```python
from build123d import *

# Parameters (mm, degrees)
F0_R     = 133.35
F1_DEPTH = 355.6
F2_W     = 101.6
F2_H     = 203.2
F3_DEPTH = 304.8
F4_R     = 127
F5_DEPTH = 355.601


with BuildPart() as f1:
    # F0 (on Front) → F1 (new body)
    with BuildSketch(Plane.XZ):
        Circle(F0_R)
    extrude(amount=F1_DEPTH)

    # F2 (on Top) → F3 (join)
    with BuildSketch(Plane.XY):
        with Locations((0, -203.2)):
            Rectangle(F2_W, F2_H)
    extrude(amount=F3_DEPTH)

    # F4 (on face) → F5 (cut, through all)
    with BuildSketch(Plane.XZ.offset(355.6)):
        Circle(F4_R)
    extrude(amount=-F5_DEPTH, mode=Mode.SUBTRACT)


solid = f1.part
```
Build history of the part. All positions in model axes, mm. A direction names the side the tool comes from. Coordinates: 2 decimals unless noted, no trailing zeros. Order: outer loops, then holes, each group sorted by start corner. A loop starts at its lowest first (then second) coordinate and runs counter-clockwise, first axis right, second up.
Item 1: Drop flat-ended pins along their axis: pin 1 Ø1.5 at (y, z) = (-70.5, 9.5) entering from +X; pin 2 Ø2 at (y, z) = (-200, -76) entering from +X; pin 3 Ø4 at (y, z) = (-196.5, -78) entering from -X. Give the stop position or say it passes through.
Filled in:
pin 1: stops at x = 133.06
pin 2: stops at x = 110.26
pin 3: stops at x = -109.57
Item 2: Saw through at B-B on z = -95. List the corners of the cut face in (x, y).
Filled in:
outline: (-93.58, -355.6) - (-84.29, -355.6) - (-84.29, 0) - (-93.58, 0) - close; (84.29, -355.6) - (93.58, -355.6) - (93.58, 0) - (84.29, 0) - close
Item 3: Mould opens along Z. For faces 4 (the cylindrical face through (-28.91, -175.31, -130.18)), 5 (the flat face through (-1, -304.8, 213)), 6 (the cylindrical face through (-27.53, -180.29, -123.98)), 7 (the flat face through (-1, -202, 304.8)) say: released by +Z, released by -Z, zero draft, split by the parting line, or undercut.
Filled in:
face 4: split by the parting line
face 5: zero draft
face 6: undercut
face 7: released by +Z
Item 4: Saw through at D-D on z = 0. List the corners of the cut face in (x, y), then the cut area to 3 significant figures.
Filled in:
outline: (-133.35, -355.6) - (-127, -355.6) - (-127, 0) - (-133.35, 0) - close; (127, -355.6) - (133.35, -355.6) - (133.35, 0) - (127, 0) - close
area: 4,520 mm2
Item 5: Drill centre lines: L1, parallel to Z at x = 0, y = -93; L2, parallel to Z at x = 0, y = -114.5; L3, parallel to Y at x = 25, z = 269. Where is each one in solid material? Low to high.
Filled in:
L1: z = -133.35 to -127, 127 to 133.35
L2: z = -133.35 to -127, 127 to 304.8
L3: y = -304.8 to -101.6
Item 6: Tool access for faces 1 (the flat face through (-50.8, -205, 213)), 2 (the flat face through (50.8, -205, 213)), 3 (the flat face through (118, -355.6, -49)): list every direction of +Z, -Z, +X, -X, +Y, -Y with a clear straight run to the whole face (end or side of a thin tool).
Filled in:
face 1: +Z, -X, +Y, -Y
face 2: +Z, +X, +Y, -Y
face 3: +Z, -Z, +X, -X, -Y
Item 7: Saw through at A-A on x = 0. List the corners of the cut face in (y, z), then the cut area to 3 significant figures.
Filled in:
outline: (-355.6, -133.35) - (0, -133.35) - (0, -127) - (-355.6, -127) - close; (-355.6, 127) - (0, 127) - (0, 133.35) - (-101.6, 133.35) - (-101.6, 304.8) - (-304.8, 304.8) - (-304.8, 133.35) - (-355.6, 133.35) - close
area: 39,400 mm2
Item 8: Saw through at C-C on y = -125.5. List the corners of the cut face in (x, z).
Filled in:
outline: (-50.8, 123.29) arc R133.35 ccw (long way) to (50.8, 123.29) - (50.8, 304.8) - (-50.8, 304.8) - close; hole circle Ø254 at (0, 0)
